For this review, take the finished solid that the model builds, in its own axes (mm). Face numbers are marked on the shaded views. A direction names the side the tool comes from. Round coordinates to 2 decimals unless told otherwise and drop trailing zeros. Write each loop counter-clockwise with the first axis right and the second up, starting at its lowest first coordinate (ties: lowest second). Pieces come first, ordered by that corner, then holes. Notation, with made-up numbers: (10, 88.25) -> (19, 88.25) arc R18 cw to (19, 97.25) -> close; hole circle Ø3 at (-17, -14.75). An arc over 180 degrees is marked (long way). Answer in a Markdown table with one row per item.
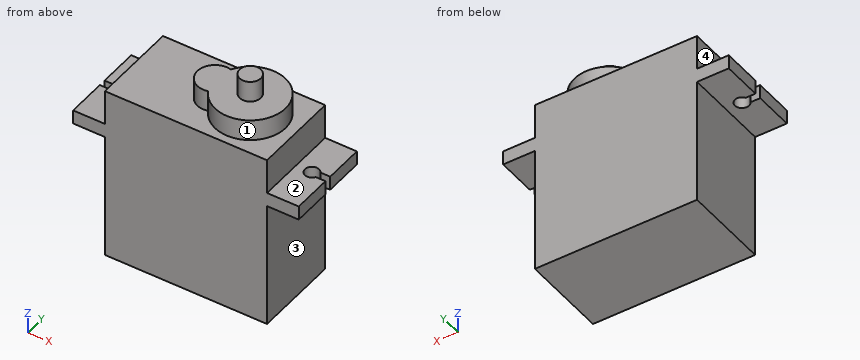
from build123d import *

# Parameters (mm, degrees)
SKETCH_1_W          = 23
SKETCH_1_H          = 12.3
EXTRUDE_1_DEPTH     = 25
SKETCH_3_R          = 5
SKETCH_3_R_2        = 2.5
EXTRUDE_2_DEPTH     = 3
SKETCH_4_R          = 1.5
EXTRUDE_3_DEPTH     = 3
EXTRUDE_START       = -5
SKETCH_5_W          = 4.5
SKETCH_5_H          = 12.3
EXTRUDE_4_DEPTH     = 2
SKETCH_6_R          = 1
CUT_EXTRUDE_1_DEPTH = 3
SKETCH_7_W          = 1.383974596
SKETCH_7_H          = 1
CUT_EXTRUDE_2_DEPTH = 10


with BuildPart() as part:
    # 草图1 → 凸台-拉伸1 (new body)
    with BuildSketch(Plane.XY):
        Rectangle(SKETCH_1_W, SKETCH_1_H)
    extrude(amount=EXTRUDE_1_DEPTH)

    # 草图3 → 凸台-拉伸2 (add)
    with BuildSketch(Plane.XY.offset(25)):
        with Locations((5, 0)):
            Circle(SKETCH_3_R)
        Circle(SKETCH_3_R_2)
    extrude(amount=EXTRUDE_2_DEPTH)

    # 草图4 → 凸台-拉伸3 (add)
    with BuildSketch(Plane.XY.offset(28)):
        with Locations((5, 0)):
            Circle(SKETCH_4_R)
    extrude(amount=EXTRUDE_3_DEPTH)

    # 草图5 → 凸台-拉伸4 (add)
    with BuildSketch(Plane.XY.offset(25).offset(EXTRUDE_START)):
        with Locations((-13.75, 0)):
            Rectangle(SKETCH_5_W, SKETCH_5_H)
        with Locations((13.75, 0)):
            Rectangle(SKETCH_5_W, SKETCH_5_H)
    extrude(amount=-EXTRUDE_4_DEPTH)

    # 草图6 → 切除-拉伸1 (cut)
    with BuildSketch(Plane.XY.offset(20)):
        with Locations((-13.75, 0)):
            Circle(SKETCH_6_R)
        with Locations(Location((13.75, 0, 0), (0, 0, 180))):
            Circle(SKETCH_6_R)
    extrude(amount=-CUT_EXTRUDE_1_DEPTH, mode=Mode.SUBTRACT)

    # 草图7 → 切除-拉伸2 (cut)
    with BuildSketch(Plane.XY.offset(20)):
        with Locations((-15.308012702, 0)):
            Rectangle(SKETCH_7_W, SKETCH_7_H)
        with Locations((15.308012702, 0)):
            Rectangle(SKETCH_7_W, SKETCH_7_H)
    extrude(amount=-CUT_EXTRUDE_2_DEPTH, mode=Mode.SUBTRACT)


solid = part.part
1) For line 1 (Y direction, x = -13.75, z = 18.4); line 2 (Z direction, x = 9.5, y = 1.5); line 3 (X direction, y = 0, z = 19.2), list the stretches that pass through material, from the lowest coordinate up. Write a range as [from, to].
Solved:
| item | result |
|---|---|
| line 1 | [-6.15, -1], [1, 6.15] |
| line 2 | [0, 28] |
| line 3 | [-12.75, 12.75] |
2) Clearance check with flat-ended pins moving along their axes: pin 1 Ø1.3 at (x, y) = (-15, 1) entering from +Z; pin 2 Ø6 at (x, y) = (0, -2.5) entering from +Z; pin 3 Ø1.5 at (y, z) = (-3.5, 16.5) entering from +X. State where each tip first meets the part, or that it passes through.
Solved:
| item | result |
|---|---|
| pin 1 | z = 20 |
| pin 2 | z = 28 |
| pin 3 | x = 11.5 |
3) Consider section C-C on y = 0. State the section outline as (x, z) points, then the cut area to 4 significant figures.
Solved:
| item | result |
|---|---|
| outline | (-12.75, 18) -> (-11.5, 18) -> (-11.5, 0) -> (11.5, 0) -> (11.5, 18) -> (12.75, 18) -> (12.75, 20) -> (11.5, 20) -> (11.5, 25) -> (10, 25) -> (10, 28) -> (6.5, 28) -> (6.5, 31) -> (3.5, 31) -> (3.5, 28) -> (-2.5, 28) -> (-2.5, 25) -> (-11.5, 25) -> (-11.5, 20) -> (-12.75, 20) -> close |
| area | 626.5 mm² |
4) For the marked faces 1, 2, 3 and 4, list the 3-axis set-ups (+Z, -Z, +X, -X, +Y, -Y) from which the entire face can be reached by the end or side of a thin tool; tool diameter is ignored.
Solved:
| item | result |
|---|---|
| face 1 | +Z |
| face 2 | +Z, +X, +Y, -Y |
| face 3 | -Z, +X, +Y, -Y |
| face 4 | +Z, -X, +Y, -Y |
5) Consider section B-B on x = 5. State the section outline as (y, z) points.
Solved:
| item | result |
|---|---|
| outline | (-6.15, 0) -> (6.15, 0) -> (6.15, 25) -> (5, 25) -> (5, 28) -> (1.5, 28) -> (1.5, 31) -> (-1.5, 31) -> (-1.5, 28) -> (-5, 28) -> (-5, 25) -> (-6.15, 25) -> close |
6) Consider section A-A on x = -13.75. State the section outline as (y, z) points.
Solved:
| item | result |
|---|---|
| outline | (-6.15, 18) -> (-1, 18) -> (-1, 20) -> (-6.15, 20) -> close; (1, 18) -> (6.15, 18) -> (6.15, 20) -> (1, 20) -> close |
7) Consider section D-D on z = 16.5. State the section outline as (x, y) points, then the cut area to 3 significant figures.
Solved:
| item | result |
|---|---|
| outline | (-11.5, -6.15) -> (11.5, -6.15) -> (11.5, 6.15) -> (-11.5, 6.15) -> close |
| area | 283 mm² |
